from build123d import *

# Parameters (mm, degrees)
F0_R     = 42
F0_R_2   = 3.2723941489
F0_R_3   = 15
F0_R_4   = 8.75
F1_DEPTH = 25
F0_R_5   = 5
F2_DEPTH = 25
F7_DEPTH = 24


# Not quite as in the source:
# - the program builds the solid bodies; features that only make, move or delete a surface that nothing else refers to are left out


with BuildPart() as f1:
    # F0 (on Front) → F1 (new body)
    with BuildSketch(Plane.XZ):
        Circle(F0_R)
        with Locations((-23.6904930325, -25.7949024873)):
            Circle(F0_R_2, mode=Mode.SUBTRACT)
        with Locations((-0.0140495196, -35.0812149592)):
            Circle(F0_R_2, mode=Mode.SUBTRACT)
        with Locations((25.8215879073, -23.6839220737)):
            Circle(F0_R_2, mode=Mode.SUBTRACT)
        with Locations((-35.0852801235, 0.0172716529)):
            Circle(F0_R_2, mode=Mode.SUBTRACT)
        with Locations((-25.8480679978, 23.7130210266)):
            Circle(F0_R_2, mode=Mode.SUBTRACT)
        with Locations((-0.0057062035, 35.0350632497)):
            Circle(F0_R_2, mode=Mode.SUBTRACT)
        Circle(F0_R_3, mode=Mode.SUBTRACT)
        with Locations((35.0598417296, 0.0224386821)):
            Circle(F0_R_2, mode=Mode.SUBTRACT)
        with Locations((25.9556279527, 23.5858062447)):
            Circle(F0_R_2, mode=Mode.SUBTRACT)
        Circle(F0_R_3)
        Circle(F0_R_4, mode=Mode.SUBTRACT)
    extrude(amount=F1_DEPTH)

    # F0 (on Front) → F2 (join)
    with BuildSketch(Plane.XZ):
        Circle(F0_R_4)
        Circle(F0_R_5, mode=Mode.SUBTRACT)
    extrude(amount=F2_DEPTH)

    # F7 (add): a face of the model
    f7_faces = [f1.faces().sort_by_distance(p)[0] for p in [
        (-40.8120606076, -25, 0),
    ]]
    extrude(f7_faces, amount=-F7_DEPTH)


solid = f1.part
Could you check a few things on this model? Use its own coordinates, in mm. Coordinates: 2 decimals unless noted, no trailing zeros. Order: outer loops, then holes, each group sorted by start corner. A loop starts at its lowest first (then second) coordinate and runs counter-clockwise, first axis right, second up.
Q1. Please list where these lines run through material, in increasing order: L1, parallel to Z at x = 0, y = -0.8; L2, parallel to X at y = -10, z = -25; L3, parallel to X at y = -17.5, z = 24.
Q2. Suppose I cut it at B-B on x = 0. Please give me the cut outline in (y, z).
Q3. Will these pins go through, and if not, where does the flat tip stop? pin 1 (5 mm diameter, centred on x = -0.01, z = -35.08, fed in from +Y); pin 2 (1 mm diameter, centred on y = -11, z = -26.5, fed in from +X); pin 3 (1 mm diameter, centred on x = -29.5, y = -20.5, fed in from +Z); pin 4 (3 mm diameter, centred on x = 23.5, y = -16.5, fed in from -Z).
Q4. Suppose I cut it at A-A on z = -33.5. Please give me the cut outline in (x, y).
Q5. Suppose I cut it at C-C on y = -15. Give the number of separate pieces and of enclosed holes in the cut face, and give its area (3 significant figures).
Q6. Suppose I cut it at D-D on x = 24. Please give me the cut outline in (y, z).
Answer:
1. L1: z = -42 to -38.35, -31.81 to -5, 5 to 31.76, 38.31 to 42
1. L2: x = -33.75 to -26.86, -20.52 to 22.83, 28.82 to 33.75
1. L3: x = -34.47 to -29.11, -22.59 to 22.71, 29.2 to 34.47
2. outline: (-25, -42) - (0, -42) - (0, -38.35) - (-25, -38.35) - close; (-25, -31.81) - (0, -31.81) - (0, -5) - (-25, -5) - close; (-25, 5) - (0, 5) - (0, 31.76) - (-25, 31.76) - close; (-25, 38.31) - (0, 38.31) - (0, 42) - (-25, 42) - close
3. pin 1: passes through
3. pin 2: stops at x = 32.98
3. pin 3: stops at z = 30.38
3. pin 4: stops at z = -35.78
4. outline: (-25.33, -25) - (-2.88, -25) - (-2.88, 0) - (-25.33, 0) - close; (2.85, -25) - (25.33, -25) - (25.33, 0) - (2.85, 0) - close
5. separate pieces: 1
5. enclosed holes: 9
5. area: 5,190 mm2
6. outline: (-25, -34.47) - (0, -34.47) - (0, -26.4) - (-25, -26.4) - close; (-25, -20.97) - (0, -20.97) - (0, 20.96) - (-25, 20.96) - close; (-25, 26.21) - (0, 26.21) - (0, 34.47) - (-25, 34.47) - close
